The figure shows three views and two pictorial views of one solid part (mm, origin at its lowest corner). Answer the questions. Give positions to 0.01 mm unless a question says otherwise; leave off trailing zeros. Order: outer loops, then holes, each group sorted by start corner. A loop starts at its lowest first (then second) coordinate and runs counter-clockwise, first axis right, second up. Notation, with made-up numbers: (20.25, 39.25) - (28.25, 39.25) arc R11 ccw to (28.25, 57.25) - close; hole circle Ø8 at (65.25, 13). An arc over 180 degrees is marked (long way). Use a Markdown table: item, result. Add a question column.
1. A flat-ended cylindrical pin translates along its axis: P1, Ø6.5, axis at x = 65, z = 10, coming from the -Y side. Find the tip coordinate at first contact, or state that the pin passes through.
2. A cutting plane is placed at C-C on x = 86.5. Determine the outline of the cut face in (y, z), and give its area (3 significant figures).
3. A cutting plane is placed at B-B on y = 6. State how many separate pieces and enclosed holes the cut face has, and give its area (3 significant figures).
4. A cutting plane is placed at A-A on x = 25. Determine the outline of the cut face in (y, z).
5. Consider L1, parallel to Z at x = 84.5, y = 5; L2, parallel to Z at x = 168.5, y = 4. Determine where each line is inside the solid, lowest interval first.
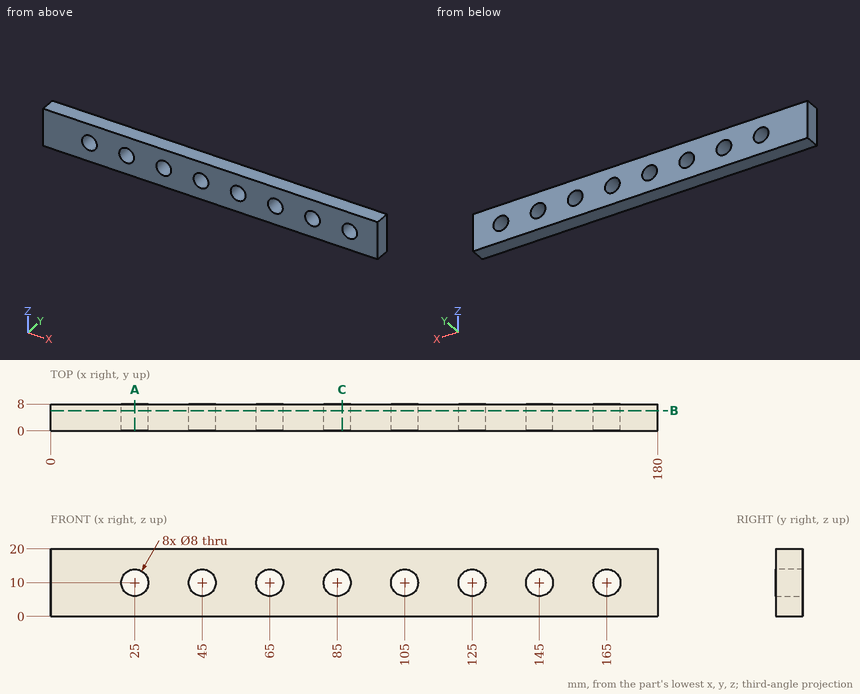
Output values:
| question | item | result |
|---|---|---|
| 1 | P1 | through |
| 2 | outline | (0, 0) - (8, 0) - (8, 6.29) - (0, 6.29) - close; (0, 13.71) - (8, 13.71) - (8, 20) - (0, 20) - close |
| 2 | area | 101 mm² |
| 3 | separate pieces | 1 |
| 3 | enclosed holes | 8 |
| 3 | area | 3,200 mm² |
| 4 | outline | (0, 0) - (8, 0) - (8, 6) - (0, 6) - close; (0, 14) - (8, 14) - (8, 20) - (0, 20) - close |
| 5 | L1 | 0 to 6.03, 13.97 to 20 |
| 5 | L2 | 0 to 8.06, 11.94 to 20 |
